from build123d import *

# Parameters (mm, degrees)
F1_DEPTH = 77.724


with BuildPart() as f1:
    # F0 (on Front) → F1 (new body)
    with BuildSketch(Plane.XZ):
        with BuildLine():
            Line((-6.8313151013, 83.892121911), (-148.7048715353, 83.892121911))
            Line((-148.7048715353, 83.892121911), (-150.2486616373, -84.8236903548))
            Line((-150.2486616373, -84.8236903548), (149.2570340633, -84.8236903548))
            Line((149.2570340633, -84.8236903548), (149.2570340633, 83.892121911))
            Line((149.2570340633, 83.892121911), (6.8313151013, 83.892121911))
            ThreePointArc((6.8313151013, 83.892121911), (61.8851573502, 57.0506992463), (84.169798531, 0))
            ThreePointArc((84.169798531, 0), (-57.0506992463, -61.8851573502), (-6.8313151013, 83.892121911))
        make_face()
        with BuildLine():
            ThreePointArc((6.8313151013, 83.892121911), (0, 84.169798531), (-6.8313151013, 83.892121911))
            Line((-6.8313151013, 83.892121911), (6.8313151013, 83.892121911))
        make_face()
        with BuildLine():
            Line((6.8313151013, 83.892121911), (-6.8313151013, 83.892121911))
            ThreePointArc((-6.8313151013, 83.892121911), (-57.0506992463, -61.8851573502), (84.169798531, 0))
            ThreePointArc((84.169798531, 0), (61.8851573502, 57.0506992463), (6.8313151013, 83.892121911))
        make_face()
    extrude(amount=F1_DEPTH)


solid = f1.part
CAD build for the part. Positions are in the model's coordinates, mm. A direction names the side the tool comes from. Give positions to 0.01 mm unless a question says otherwise; leave off trailing zeros. Put each result on its own line as item: value. Start each with the question number.
(1) Probe L1, parallel to Z at x = -35, y = -54; L2, parallel to X at y = -42, z = 42; L3, parallel to X at y = -16, z = -59. List the from-to ranges inside material, lowest first.
(2) Which spindle directions (+Z, -Z, +X, -X, +Y, -Y) get a long thin tool onto all of the face, cutting with end or side? Do faces 1 (the face through (0.1, -38.32, 84.17)), 2 (the face through (-77, -38, 83.892)), 3 (the face through (79, -38, 83.892)). Say none if no direction does.
(3) Flat gauge pins, fed straight in: pin 1 Ø23.5 at (x, y) = (-93.5, -45.5) entering from +Z; pin 2 Ø1.5 at (x, z) = (-2, 0) entering from +Y. Where does each tip first touch, or does it go through?
Response values:
1. L1: z = -84.82 to 83.89
1. L2: x = -149.09 to 149.26
1. L3: x = -150.01 to 149.26
2. face 1: +Z, +Y, -Y
2. face 2: +Z, -X, +Y, -Y
2. face 3: +Z, +X, +Y, -Y
3. pin 1: stops at z = 83.89
3. pin 2: stops at y = 0
